Input: part model. Units: mm. Frame: model coordinates. A direction names the side the tool comes from. Give positions to 0.01 mm unless a question says otherwise; leave off trailing zeros. Loops run counter-clockwise (first coordinate to the right, second up) from the corner with the lowest first, then second, coordinate; pieces in that order, holes last.
from build123d import *

# Parameters (mm, degrees)
BOSS_EXTRUDE1_DEPTH       = 19.5
SKETCH2_R                 = 5.25
HOBB_CLEARANCE_DEPTH      = 22
M3_CLEARANCE_HOLE1_D      = 3.6
SKETCH6_R                 = 12
CUT_EXTRUDE2_DEPTH        = 22
CUT_EXTRUDE3_START        = 15.5
CUT_EXTRUDE3_DEPTH        = 15.5
M3X0_5_TAPPED_HOLE1_D     = 2.5
FILLET1_R                 = 1
M5X0_8_TAPPED_HOLE1_D     = 4.2
M5X0_8_TAPPED_HOLE1_DEPTH = 21
M5X0_8_TAPPED_HOLE1_TIP   = 1.2618073
SKETCH12_R                = 1
CUT_EXTRUDE4_DEPTH        = 51.845353932
BOSS_EXTRUDE2_DEPTH       = 15
BOSS_EXTRUDE2_DEPTH_BACK  = 0.005
SKETCH14_W                = 42
SKETCH14_H                = 19.5
SKETCH15_R                = 1
CUT_EXTRUDE6_DEPTH        = 26.51413021
CUT_EXTRUDE7_START        = -2
CUT_EXTRUDE7_DEPTH        = 11
M3X0_5_TAPPED_HOLE2_D     = 2.5
FILLET3_R                 = 2
CHAMFER2_SIZE             = 1
CHAMFER2_SIZE2            = 1.732050808
FILLET4_START             = -1
FILLET4_DEPTH             = 16.5


with BuildPart() as part:
    # Sketch1 → Boss-Extrude1 (new body)
    with BuildSketch(Plane.XY):
        Polygon((21, -21), (21, 31), (14, 31), (14, 21), (-21, 21), (-21, -21), align=None)
    extrude(amount=BOSS_EXTRUDE1_DEPTH)

    # Sketch2 → Hobb Clearance (cut)
    with BuildSketch(Plane.XY.offset(19.5)):
        Circle(SKETCH2_R)
    extrude(amount=-HOBB_CLEARANCE_DEPTH, mode=Mode.SUBTRACT)

    # M3 Clearance Hole1 (through all)
    with Locations(Plane.XY.offset(19.5)):
        with Locations((-15.5, 15.5), (15.5, 15.5), (15.5, -15.5), (-15.5, -15.5)):
            Hole(M3_CLEARANCE_HOLE1_D / 2)

    # Sketch6 → Cut-Extrude2 (cut)
    with BuildSketch(Plane.XY.offset(19.5)):
        with Locations((16.1475, 0)):
            Circle(SKETCH6_R)
    extrude(amount=-CUT_EXTRUDE2_DEPTH, mode=Mode.SUBTRACT)

    # Sketch7 → Cut-Extrude3 (cut)
    with BuildSketch(Plane.XY.offset(CUT_EXTRUDE3_START)):
        with BuildLine():
            Line((21, -10.975119305), (21, -21))
            Line((21, -21), (12, -21))
            Line((12, -21), (12, -11.260472626))
            ThreePointArc((12, -11.260472626), (16.527780001, -11.99397295), (21, -10.975119305))
        make_face()
    extrude(amount=-CUT_EXTRUDE3_DEPTH, mode=Mode.SUBTRACT)

    # M3x0.5 Tapped Hole1 (through all)
    with Locations(Plane.ZY.offset(-14)):
        with Locations((9.75, 26)):
            Hole(M3X0_5_TAPPED_HOLE1_D / 2)

    # Fillet1
    fillet1_edges = [part.edges().sort_by_distance(p)[0] for p in [
        (4.468315722, -2.756202933, 9.75),
        (4.468315722, 2.756202933, 9.75),
    ]]
    fillet(fillet1_edges, radius=FILLET1_R)

    # M5x0.8 Tapped Hole1
    with Locations(Plane(origin=(0, 21, 0), x_dir=(1, 0, 0), z_dir=(0, 1, 0))):
        with Locations((4.191547948, -9.75)):
            Hole(M5X0_8_TAPPED_HOLE1_D / 2, depth=M5X0_8_TAPPED_HOLE1_DEPTH)
            with Locations((0, 0, -(M5X0_8_TAPPED_HOLE1_DEPTH + M5X0_8_TAPPED_HOLE1_TIP / 2))):  # 118° drill point
                Cone(0, M5X0_8_TAPPED_HOLE1_D / 2, M5X0_8_TAPPED_HOLE1_TIP, mode=Mode.SUBTRACT)

    # Sketch12 → Cut-Extrude4 (cut, through all)
    with BuildSketch(Plane(origin=(0, 21, 0), x_dir=(1, 0, 0), z_dir=(0, 1, 0))):
        with Locations(Location((4.191547948, -9.75, 0), (0, 0, 270))):
            Circle(SKETCH12_R)
    extrude(amount=-CUT_EXTRUDE4_DEPTH, mode=Mode.SUBTRACT)

    # Sketch14 → Boss-Extrude2 (add, two sides: drawn at the far end of the back side and taken through both)
    with BuildSketch(Plane.XZ.offset(21).offset(-BOSS_EXTRUDE2_DEPTH_BACK)):
        with Locations((0, 9.75)):
            Rectangle(SKETCH14_W, SKETCH14_H)
    extrude(amount=BOSS_EXTRUDE2_DEPTH + BOSS_EXTRUDE2_DEPTH_BACK)

    # Sketch15 → Cut-Extrude6 (cut)
    with BuildSketch(Plane(origin=(0, -20.995, 0), x_dir=(1, 0, 0), z_dir=(0, 1, 0))):
        with Locations(Location((4.191547948, -9.75, 0), (0, 0, 322.12020771))):
            Circle(SKETCH15_R)
    extrude(amount=-CUT_EXTRUDE6_DEPTH, mode=Mode.SUBTRACT)

    # Sketch16 → Cut-Extrude7 (cut)
    with BuildSketch(Plane(origin=(0, -20.995, 0), x_dir=(1, 0, 0), z_dir=(0, 1, 0)).offset(CUT_EXTRUDE7_START)):
        Polygon((-17.558452052, -1.75), (-9.058452052, -1.75), (-9.058452052, -3.75), (-8.058452052, -3.75), (-2.558452052, -3.75), (-2.558452052, -12.75), (2.691547948, -12.75), (5.691547948, -12.75), (10.941547948, -12.75), (10.941547948, -3.75), (16.441547948, -3.75), (17.441547948, -3.75), (17.441547948, 0), (-17.558452052, 0), (-17.558452052, -0.75), align=None)
    extrude(amount=-CUT_EXTRUDE7_DEPTH, mode=Mode.SUBTRACT)

    # M3x0.5 Tapped Hole2 (through all)
    with Locations(Plane(origin=(0, 0, 3.75), x_dir=(-1, 0, 0), z_dir=(0, 0, -1))):
        with Locations((5.333452052, -28.495), (-13.716547948, -28.495)):
            Hole(M3X0_5_TAPPED_HOLE2_D / 2)

    # Chamfer1: read off the stored shape, not the designer's step
    # Chamfer1 outline → Chamfer1 (revolve, cut)
    with BuildSketch(Plane(origin=(4.191547948, 0, 9.75), x_dir=(1, 0, 0), z_dir=(0, 0, 1))):
        Polygon((3, -22.995), (1, -19.530898385), (1, -22.995), align=None)
    revolve(axis=Axis((4.191547948, 0, 9.75), (0, 1, 0)), mode=Mode.SUBTRACT)

    # Fillet3
    fillet3_edges = [part.edges().sort_by_distance(p)[0] for p in [
        (21, -20.995, 7.75),
        (12, -20.995, 7.75),
        (-21, -36, 9.75),
        (21, -36, 9.75),
        (-21, 21, 9.75),
        (21, 10.975119305, 9.75),
        (21, -10.975119305, 17.5),
        (12, -11.260472626, 7.75),
        (14, 31, 9.75),
        (21, 31, 9.75),
        (14, 21, 9.75),
    ]]
    fillet(fillet3_edges, radius=FILLET3_R)

    # Chamfer2
    chamfer2_edges = [part.edges().sort_by_distance(p)[0] for p in [
        (3.40224726, -36, 9.135993141),
    ]]
    chamfer2_side = [part.faces().sort_by_distance(p)[0] for p in [
        (3.40224726, -34.9975, 9.135993141),
    ]]
    chamfer(chamfer2_edges, length=CHAMFER2_SIZE, length2=CHAMFER2_SIZE2, reference=chamfer2_side[0])

    # Fillet4: read off the stored shape, not the designer's step
    # Fillet4 outline → Fillet4 (cut)
    with BuildSketch(Plane.XY.offset(FILLET4_START)):
        with BuildLine():
            ThreePointArc((9.106973684, -9.717560867), (11.234934474, -12.204064485), (12, -15.386138039))
            Line((12, -15.386138039), (12, -12.578085854))
            ThreePointArc((12, -12.578085854), (11.696530072, -11.518941995), (10.878214286, -10.781216446))
            ThreePointArc((10.878214286, -10.781216446), (9.969659856, -10.28757946), (9.106973684, -9.717560867))
        make_face()
    extrude(amount=FILLET4_DEPTH, mode=Mode.SUBTRACT)


solid = part.part
(1) Pin query (flat end, axial travel): pin 1 Ø1.5 at (x, y) = (-10, 23.5) entering from -Z; pin 2 Ø1 at (x, z) = (8, 9.5) entering from +Y; pin 3 Ø7 at (x, y) = (-5, -29) entering from -Z; pin 4 Ø5 at (y, z) = (26, 5.5) entering from -X. Return the tip coordinate at first contact, or that it passes through.
Values follow:
pin 1: passes through
pin 2: stops at y = 21
pin 3: stops at z = 3.75
pin 4: stops at x = 14
(2) Reachability of faces 1 (the cylindrical face through (10.547, 10.613, 9.886)), 2 (the cylindrical face through (12.601, -20.425, 7.642)), 3 (the flat face through (-2.558, -28, 8)) from +Z, -Z, +X, -X, +Y, -Y: full face, straight path, thin tool, end or side. Return the list, or none.
Values follow:
face 1: +Z, -Z
face 2: -Z, +X
face 3: -Z
(3) Cut plane B-B (y = 26). Return the cut outline in (x, z).
Values follow:
outline: (14, 0) - (21, 0) - (21, 8.5) - (14, 8.5) - close; (14, 11) - (21, 11) - (21, 19.5) - (14, 19.5) - close
(4) Cut plane C-C (y = -16.5). Return the cut outline in (x, z), and give its area (3 significant figures).
Values follow:
outline: (-21, 0) - (-17, 0) - (-17, 19.5) - (-21, 19.5) - close; (-14, 0) - (12, 0) - (12, 15.5) - (14, 15.5) - (14, 19.5) - (-14, 19.5) - close; (17, 15.5) - (21, 15.5) - (21, 19.5) - (17, 19.5) - close; hole circle Ø2 at (4.19, 9.75)
area: 606 mm2
(5) Mould query, pull axis Y, two halves, no side actions, for faces 4 (the cylindrical face through (20.4, -35.43, 9.89)), 5 (the flat face through (-21, -7, 10)), 6 (the cylindrical face through (13.4, 21.57, 9.89)), 7 (the flat face through (4, -28, 12.75)). Classes: +Y half, -Y half, draft (parallel to the pull), parting line (faces both ways), or undercut.
Values follow:
face 4: -Y half
face 5: draft
face 6: +Y half
face 7: undercut
(6) Ray query, probe 1 along Y at (x, z) = (-15.5, 5.75); probe 2 along Y at (x, z) = (-2, 7.75) (3 decimals); probe 3 along X at (y, z) = (-34.2, 9.75). Return the intervals inside material, ascending.
Values follow:
probe 1: y = -36 to -17.3, -13.7 to 13.7, 17.3 to 21
probe 2: y = -36 to -33.995, -22.995 to -4.854, 4.854 to 21
probe 3: x = -20.99 to 3.19, 5.19 to 20.99
(7) Cut plane A-A (x = 0). Return the cut outline in (y, z) (3 decimals), and give its area (4 significant figures).
Values follow:
outline: (-36, 0) - (-33.995, 0) - (-33.995, 12.75) - (-22.995, 12.75) - (-22.995, 0) - (-5.25, 0) - (-5.25, 19.5) - (-36, 19.5) - close; (5.25, 0) - (21, 0) - (21, 19.5) - (5.25, 19.5) - close
area: 766.5 mm2
(8) Cut plane D-D (x = -15.5). Return the cut outline in (y, z) (3 decimals), and give its area (3 significant figures).
Values follow:
outline: (-36, 0) - (-33.995, 0) - (-33.995, 1.75) - (-22.995, 1.75) - (-22.995, 0) - (-17.3, 0) - (-17.3, 19.5) - (-36, 19.5) - close; (-13.7, 0) - (13.7, 0) - (13.7, 19.5) - (-13.7, 19.5) - close; (17.3, 0) - (21, 0) - (21, 19.5) - (17.3, 19.5) - close
area: 952 mm2
